Can you work these out from the model? Positions are in its coordinate system, mm. Give positions to 0.01 mm unless a question says otherwise; leave off trailing zeros. Loops run counter-clockwise (first coordinate to the right, second up) from the corner with the lowest first, then second, coordinate; pieces in that order, holes last. Notation, with made-up numbers: M 84.5,46 L 143.5,46 A11 cw 143.5,59 Z; hole C 80.25,41 d1. An arc over 180 degrees is marked long. Put each result on its own line as item: value. Start each with the question number.
1) Please list where these lines run through material, in increasing order: line 1 along X through (y, z) = (4.05, 0); line 2 along X through (y, z) = (2.45, 2.5); line 3 along X through (y, z) = (3.55, 16.5). Write a range as from..to.
2) For P1, Ø9, axis at x = -50, z = -16, coming from the -Y side, with a flat end and sliding along its axis, tell me the tip position at first contact or that it passes through.
3) Imagine slicing it at C-C (y = 4.7). State how many separate pieces and enclosed holes the cut face has, then the cut area to 3 significant figures.
4) Imagine slicing it at A-A (x = 0). Write out the boundary of the cut face in (y, z), then the cut area to 3 significant figures.
5) Imagine slicing it at D-D (x = 15.5). Write out the boundary of the cut face in (y, z), then the cut area to 3 significant figures.
6) Imagine slicing it at B-B (z = 2). Write out the boundary of the cut face in (x, y), then the cut area to 3 significant figures.
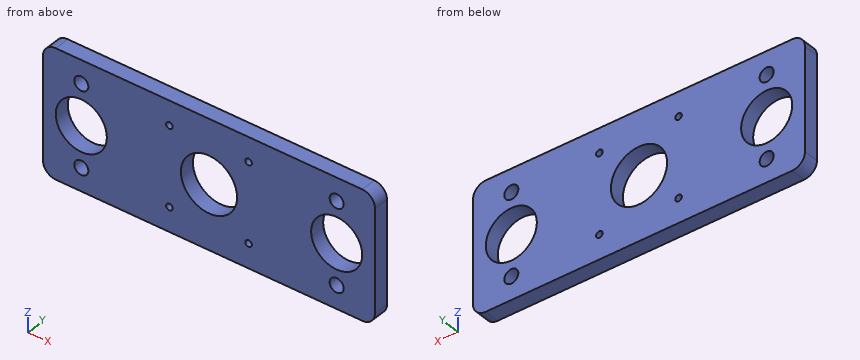
from build123d import *

# Parameters (mm, degrees)
SKETCH_1_R      = 2.75
SKETCH_1_R_2    = 11
SKETCH_1_R_3    = 1.283558174
SKETCH_1_R_4    = 10
EXTRUDE_1_DEPTH = 6


with BuildPart() as part:
    # 草图1 → 凸台-拉伸1 (new body)
    with BuildSketch(Plane(origin=(0, 0, 0), x_dir=(1, 0, 0), z_dir=(0, 1, 0))):
        with BuildLine():
            ThreePointArc((-65, 20), (-63.535533906, 23.535533906), (-60, 25))
            Line((-60, 25), (0, 25))
            Line((0, 25), (60, 25))
            ThreePointArc((60, 25), (63.535533906, 23.535533906), (65, 20))
            Line((65, 20), (65, -20))
            ThreePointArc((65, -20), (63.535533906, -23.535533906), (60, -25))
            Line((60, -25), (-60, -25))
            ThreePointArc((-60, -25), (-63.535533906, -23.535533906), (-65, -20))
            Line((-65, -20), (-65, 20))
        make_face()
        with Locations(Location((-50, 16, 0), (0, 0, 270))):
            Circle(SKETCH_1_R, mode=Mode.SUBTRACT)
        with Locations(Location((0, 0, 0), (0, 0, 270))):
            Circle(SKETCH_1_R_2, mode=Mode.SUBTRACT)
        with Locations(Location((15.5, 15.5, 0), (0, 0, 270))):
            Circle(SKETCH_1_R_3, mode=Mode.SUBTRACT)
        with Locations(Location((15.5, -15.5, 0), (0, 0, 270))):
            Circle(SKETCH_1_R_3, mode=Mode.SUBTRACT)
        with Locations(Location((-15.5, -15.5, 0), (0, 0, 270))):
            Circle(SKETCH_1_R_3, mode=Mode.SUBTRACT)
        with Locations(Location((-15.5, 15.5, 0), (0, 0, 270))):
            Circle(SKETCH_1_R_3, mode=Mode.SUBTRACT)
        with Locations(Location((50, 0, 0), (0, 0, 270))):
            Circle(SKETCH_1_R_4, mode=Mode.SUBTRACT)
        with Locations(Location((50, 16, 0), (0, 0, 270))):
            Circle(SKETCH_1_R, mode=Mode.SUBTRACT)
        with Locations(Location((50, -16, 0), (0, 0, 270))):
            Circle(SKETCH_1_R, mode=Mode.SUBTRACT)
        with Locations(Location((-50, -16, 0), (0, 0, 270))):
            Circle(SKETCH_1_R, mode=Mode.SUBTRACT)
        with Locations(Location((-50, 0, 0), (0, 0, 270))):
            Circle(SKETCH_1_R_4, mode=Mode.SUBTRACT)
    extrude(amount=EXTRUDE_1_DEPTH)


solid = part.part
Recorded:
1. line 1: -65..-60, -40..-11, 11..40, 60..65
1. line 2: -65..-59.68, -40.32..-10.71, 10.71..40.32, 59.68..65
1. line 3: -65..-52.7, -47.3..-16.3, -14.7..14.7, 16.3..47.3, 52.7..65
2. P1: y = 0
3. separate pieces: 1
3. enclosed holes: 11
3. area: 5,350 mm²
4. outline: M 0,-25 L 6,-25 L 6,-11 L 0,-11 Z; M 0,11 L 6,11 L 6,25 L 0,25 Z
4. area: 168 mm²
5. outline: M 0,-25 L 6,-25 L 6,-16.78 L 0,-16.78 Z; M 0,-14.22 L 6,-14.22 L 6,14.22 L 0,14.22 Z; M 0,16.78 L 6,16.78 L 6,25 L 0,25 Z
5. area: 269 mm²
6. outline: M -65,0 L -59.8,0 L -59.8,6 L -65,6 Z; M -40.2,0 L -10.82,0 L -10.82,6 L -40.2,6 Z; M 10.82,0 L 40.2,0 L 40.2,6 L 10.82,6 Z; M 59.8,0 L 65,0 L 65,6 L 59.8,6 Z
6. area: 415 mm²
